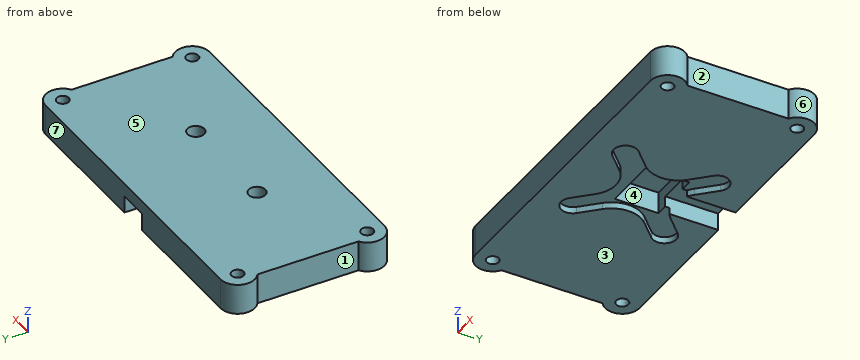
```python
from build123d import *

# Parameters (mm, degrees)
SKETCH1_R           = 1.6
BOSS_EXTRUDE1_DEPTH = 8
CUT_EXTRUDE4_DEPTH  = 1.7
CUT_EXTRUDE5_DEPTH  = 7.4
SKETCH1_9_W         = 8
SKETCH1_9_H         = 13.9
CUT_EXTRUDE6_DEPTH  = 4.5
SKETCH2_R           = 2.2
CUT_EXTRUDE11_DEPTH = 6


with BuildPart() as part:
    # Sketch1 → Boss-Extrude1 (new body)
    with BuildSketch(Plane.XY):
        with BuildLine():
            Line((-42.5, 13.258342613), (-42.5, -13.258342613))
            ThreePointArc((-42.5, -13.258342613), (-44.30624304, -18.30624304), (-40, -21.5))
            Line((-40, -21.5), (40, -21.5))
            ThreePointArc((40, -21.5), (44.30624304, -18.30624304), (42.5, -13.258342613))
            Line((42.5, -13.258342613), (42.5, 13.258342613))
            ThreePointArc((42.5, 13.258342613), (44.30624304, 18.30624304), (40, 21.5))
            Line((40, 21.5), (-40, 21.5))
            ThreePointArc((-40, 21.5), (-44.30624304, 18.30624304), (-42.5, 13.258342613))
        make_face()
        with Locations((-40, -17)):
            Circle(SKETCH1_R, mode=Mode.SUBTRACT)
        with Locations((40, -17)):
            Circle(SKETCH1_R, mode=Mode.SUBTRACT)
        with Locations((-40, 17)):
            Circle(SKETCH1_R, mode=Mode.SUBTRACT)
        with Locations((40, 17)):
            Circle(SKETCH1_R, mode=Mode.SUBTRACT)
    extrude(amount=BOSS_EXTRUDE1_DEPTH)

    # Sketch1_7 → Cut-Extrude4 (cut)
    with BuildSketch(Plane.XY):
        with BuildLine():
            Line((-5.489949494, 9.874011537), (-9.828784258, 14.212846302))
            ThreePointArc((-9.828784258, 14.212846302), (-14.212846302, 14.212846302), (-14.212846302, 9.828784258))
            Line((-14.212846302, 9.828784258), (-9.874011537, 5.489949494))
            ThreePointArc((-9.874011537, 5.489949494), (-7.6, 0), (-9.874011537, -5.489949494))
            Line((-9.874011537, -5.489949494), (-14.212846302, -9.828784258))
            ThreePointArc((-14.212846302, -9.828784258), (-14.212846302, -14.212846302), (-9.828784258, -14.212846302))
            Line((-9.828784258, -14.212846302), (-5.489949494, -9.874011537))
            ThreePointArc((-5.489949494, -9.874011537), (0, -7.6), (5.489949494, -9.874011537))
            Line((5.489949494, -9.874011537), (9.828784258, -14.212846302))
            ThreePointArc((9.828784258, -14.212846302), (14.212846302, -14.212846302), (14.212846302, -9.828784258))
            Line((14.212846302, -9.828784258), (9.874011537, -5.489949494))
            ThreePointArc((9.874011537, -5.489949494), (7.6, 0), (9.874011537, 5.489949494))
            Line((9.874011537, 5.489949494), (14.212846302, 9.828784258))
            ThreePointArc((14.212846302, 9.828784258), (14.212846302, 14.212846302), (9.828784258, 14.212846302))
            Line((9.828784258, 14.212846302), (5.489949494, 9.874011537))
            ThreePointArc((5.489949494, 9.874011537), (0, 7.6), (-5.489949494, 9.874011537))
        make_face()
    extrude(amount=CUT_EXTRUDE4_DEPTH, mode=Mode.SUBTRACT)

    # Sketch1_8 → Cut-Extrude5 (cut)
    with BuildSketch(Plane.XY):
        Polygon((-7.1, -3.85), (7.1, -3.85), (7.1, 3.85), (7.1, 7.6), (-7.1, 7.6), (-7.1, 3.85), align=None)
    extrude(amount=CUT_EXTRUDE5_DEPTH, mode=Mode.SUBTRACT)

    # Sketch1_9 → Cut-Extrude6 (cut)
    with BuildSketch(Plane.XY):
        with Locations((0, 14.55)):
            Rectangle(SKETCH1_9_W, SKETCH1_9_H)
    extrude(amount=CUT_EXTRUDE6_DEPTH, mode=Mode.SUBTRACT)

    # Sketch2 → Cut-Extrude11 (cut)
    with BuildSketch(Plane.XY.offset(8)):
        with Locations((-14, -3)):
            Circle(SKETCH2_R)
        with Locations(Location((14, -3, 0), (0, 0, 180))):
            Circle(SKETCH2_R)
    extrude(amount=-CUT_EXTRUDE11_DEPTH, mode=Mode.SUBTRACT)


solid = part.part
```
Source: CAD feature listing. Evaluate the final solid. Frame: model axes, mm. Face numbers are marked on the shaded views. A direction names the side the tool comes from. Coordinates: 2 decimals unless noted, no trailing zeros. Write each loop counter-clockwise with the first axis right and the second up, starting at its lowest first coordinate (ties: lowest second). Pieces come first, ordered by that corner, then holes. Notation, with made-up numbers: (50, 17.25) - (81, 17.25) arc R8 ccw to (81, 31.25) - close; hole circle Ø7 at (58, 6). An arc over 180 degrees is marked (long way). Answer as a JSON object with one key per item and string values.
Q1. Draft query along Y for the marked faces 5, 6 and 7. Return one class per face: released by +Y, released by -Y, zero draft, split by the parting line, or undercut.
Ans:
{"face 5": "zero draft", "face 6": "undercut", "face 7": "released by +Y"}
Q2. Section query C-C, the plane y = 17. Output: boundary loops of the cut face in (x, z), plus the area to 3 significant figures.
Ans:
{"outline": "(-44.5, 0) - (-41.6, 0) - (-41.6, 8) - (-44.5, 8) - close; (-38.4, 0) - (-4, 0) - (-4, 4.5) - (4, 4.5) - (4, 0) - (38.4, 0) - (38.4, 8) - (-38.4, 8) - close; (41.6, 0) - (44.5, 0) - (44.5, 8) - (41.6, 8) - close", "area": "625 mm2"}
Q3. First-contact query: pin 1 Ø4 at (y, z) = (5.5, 6) entering from +X; pin 2 Ø4 at (x, y) = (-14, -3) entering from +Z; pin 3 Ø2 at (y, z) = (12.5, 6.5) entering from +X. Flat tips, straight axial feed; report the tip coordinate or a pass-through.
Ans:
{"pin 1": "stops at x = 42.5", "pin 2": "stops at z = 2", "pin 3": "stops at x = 42.83"}
Q4. Section query D-D, the plane y = -9. Output: boundary loops of the cut face in (x, z), plus the area to 3 significant figures.
Ans:
{"outline": "(-42.5, 0) - (-13.38, 0) - (-13.38, 1.7) - (-4.45, 1.7) - (-4.45, 0) - (4.45, 0) - (4.45, 1.7) - (13.38, 1.7) - (13.38, 0) - (42.5, 0) - (42.5, 8) - (-42.5, 8) - close", "area": "650 mm2"}
Q5. Section query B-B, the plane z = 3.5. Output: boundary loops of the cut face in (x, y), plus the area to 3 significant figures.
Ans:
{"outline": "(-42.5, -13.26) arc R4.5 ccw to (-40, -21.5) - (40, -21.5) arc R4.5 ccw to (42.5, -13.26) - (42.5, 13.26) arc R4.5 ccw to (40, 21.5) - (4, 21.5) - (4, 7.6) - (7.1, 7.6) - (7.1, -3.85) - (-7.1, -3.85) - (-7.1, 7.6) - (-4, 7.6) - (-4, 21.5) - (-40, 21.5) arc R4.5 ccw to (-42.5, 13.26) - close; hole circle Ø3.2 at (-40, -17); hole circle Ø3.2 at (-40, 17); hole circle Ø4.4 at (-14, -3); hole circle Ø4.4 at (14, -3); hole circle Ø3.2 at (40, -17); hole circle Ø3.2 at (40, 17)", "area": "3,360 mm2"}
Q6. Section query A-A, the plane y = -17. Output: boundary loops of the cut face in (x, z).
Ans:
{"outline": "(-44.5, 0) - (-41.6, 0) - (-41.6, 8) - (-44.5, 8) - close; (-38.4, 0) - (38.4, 0) - (38.4, 8) - (-38.4, 8) - close; (41.6, 0) - (44.5, 0) - (44.5, 8) - (41.6, 8) - close"}
Q7. Set-up query: the marked faces 1, 2, 3 and 4. Return all of +Z, -Z, +X, -X, +Y, -Y with unobstructed straight access to the full face (end or side cutting, diameter ignored); none if empty.
Ans:
{"face 1": "+Z, -Z, -X", "face 2": "+Z, -Z, +X", "face 3": "-Z, +X, -X, +Y, -Y", "face 4": "-Z"}
Q8. Material intervals for line 1 (Y direction, x = 40, z = 4.75); line 2 (X direction, y = 0, z = 4); line 3 (Y direction, x = -14, z = 5.35), sorted ascending. Write a range as [from, to].
Ans:
{"line 1": "y = [-21.5, -18.6], [-15.4, 15.4], [18.6, 21.5]", "line 2": "x = [-42.5, -7.1], [7.1, 42.5]", "line 3": "y = [-21.5, -5.2], [-0.8, 21.5]"}
